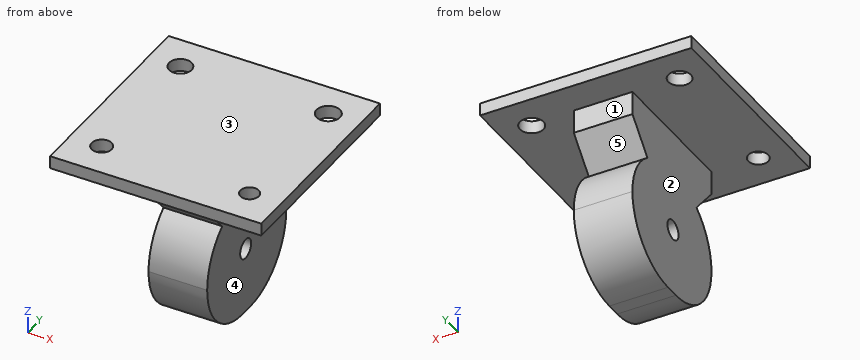
from build123d import *

# Parameters (mm, degrees)
SKETCH_W        = 50
SKETCH_H        = 50
SKETCH_R        = 2.673206
SKETCH_R_2      = 2.795993
SKETCH_R_3      = 2.184497
SKETCH_R_4      = 2.376808
PAD_DEPTH       = 3
SKETCH001_W     = 13.880783
SKETCH001_H     = 33.313887
PAD001_DEPTH    = 40
FILLET_R        = 15
POCKET_DEPTH    = 31.618891
SKETCH003_R     = 2.326985
POCKET001_DEPTH = 32.263892


with BuildPart() as part:
    # Sketch → Pad (new body)
    with BuildSketch(Plane.XY):
        Rectangle(SKETCH_W, SKETCH_H)
        with Locations((-17.5, 16.5883488719)):
            Circle(SKETCH_R, mode=Mode.SUBTRACT)
        with Locations((17.5, 16.588348)):
            Circle(SKETCH_R_2, mode=Mode.SUBTRACT)
        with Locations((17.5, -16.5883488719)):
            Circle(SKETCH_R_3, mode=Mode.SUBTRACT)
        with Locations((-17.5, -16.5883488719)):
            Circle(SKETCH_R_4, mode=Mode.SUBTRACT)
    extrude(amount=PAD_DEPTH)

    # Sketch001 (on Face9 of Pad) → Pad001 (join)
    with BuildSketch(Plane(origin=(0, 0, 0), x_dir=(1, 0, 0), z_dir=(0, 0, -1))):
        with Locations((0.3225005, -0.4243995)):
            Rectangle(SKETCH001_W, SKETCH001_H)
    extrude(amount=PAD001_DEPTH)

    # Fillet
    fillet_edges = [part.edges().sort_by_distance(p)[0] for p in [
        (0.3225, -16.232544, -40),
        (0.322501, 17.081343, -40),
    ]]
    fillet(fillet_edges, radius=FILLET_R)

    # Sketch002 (on Face1 of Fillet) → Pocket (cut, through all)
    with BuildSketch(Plane(origin=(-6.617891, 0, 0), x_dir=(0, -1, 0), z_dir=(-1, 0, 0))):
        with BuildLine():
            ThreePointArc((16.232544, -25), (14.5567914087, -18.1105565543), (9.9039532011, -12.7604468028))
            Line((9.9039532011, -12.7604468028), (16.232544, -5.5931115513))
            Line((16.232544, -5.5931115513), (16.232544, -25))
        make_face()
        with BuildLine():
            ThreePointArc((-10.7527522011, -12.7604468028), (-15.4055904087, -18.1105565543), (-17.081343, -25))
            Line((-17.081343, -5.5931115513), (-17.081343, -25))
            Line((-10.7527522011, -12.7604468028), (-17.081343, -5.5931115513))
        make_face()
    extrude(amount=-POCKET_DEPTH, mode=Mode.SUBTRACT)

    # Sketch003 (on Face18 of Pocket) → Pocket001 (cut, through all)
    with BuildSketch(Plane.YZ.offset(7.262892)):
        with Locations((0, -24.346371)):
            Circle(SKETCH003_R)
    extrude(amount=-POCKET001_DEPTH, mode=Mode.SUBTRACT)


solid = part.part
Input: part model. Units: mm. Frame: model coordinates. Face numbers are marked on the shaded views. A direction names the side the tool comes from. Round coordinates to 2 decimals unless told otherwise and drop trailing zeros. Write each loop counter-clockwise with the first axis right and the second up, starting at its lowest first coordinate (ties: lowest second). Pieces come first, ordered by that corner, then holes.
1) Cut plane B-B (y = -12.5). Return the cut outline in (x, z), then the cut area to 3 significant figures.
2) Cut plane A-A (x = 17.5). Return the cut outline in (y, z), then the cut area to 3 significant figures.
3) Draft query along Z for the marked faces 3, 4 and 5. Return one class per face: pulls with the +Z half, pulls with the -Z half, needs draft (parallel to the pull), parting line crosses it, or undercut.
4) Cut plane D-D (y = 5.5). Return the cut outline in (x, z).
5) Reachability of the marked faces 1 and 2 from +Z, -Z, +X, -X, +Y, -Y: full face, straight path, thin tool, end or side. Return the list, or none.
6) Cut plane C-C (x = -3.5). Return the cut outline in (y, z), then the cut area to 3 significant figures.
7) Contact query for flat-ended pins moving along their axis: P1, Ø10, axis at y = -4.5, z = -12, coming from the +X side; P2, Ø4.5, axis at x = -2, z = -1.5, coming from the -Y side; P3, Ø15, axis at x = -4.5, y = 11.5, coming from the -Z side; P4, Ø2, axis at x = 8.5, y = -7, coming from the -Z side. Output: stop coordinate, or through.
8) Ray query, L1, parallel to Y at x = 17.5, z = 1.75; L2, parallel to Y at x = -17.5, z = 1.1; L3, parallel to Z at x = 3.5, y = 0. Return the intervals inside material, ascending.
Geometry says:
1. outline: (-25, 0) - (-6.62, 0) - (-6.62, -9.82) - (7.26, -9.82) - (7.26, 0) - (25, 0) - (25, 3) - (-25, 3) - close; (-6.62, -34.9) - (7.26, -34.9) - (7.26, -15.1) - (-6.62, -15.1) - close
1. area: 561 mm2
2. outline: (-25, 0) - (-18.77, 0) - (-18.77, 3) - (-25, 3) - close; (-14.4, 0) - (13.79, 0) - (13.79, 3) - (-14.4, 3) - close; (19.38, 0) - (25, 0) - (25, 3) - (19.38, 3) - close
2. area: 120 mm2
3. face 3: pulls with the +Z half
3. face 4: needs draft
3. face 5: undercut
4. outline: (-25, 0) - (-6.62, 0) - (-6.62, -39.61) - (7.26, -39.61) - (7.26, 0) - (25, 0) - (25, 3) - (-25, 3) - close
5. face 1: -Z, +X, -X, +Y
5. face 2: -Z, -X, +Y, -Y
6. outline: (-25, 0) - (-16.23, 0) - (-16.23, -5.59) - (-9.9, -12.76) arc R15 ccw to (-1.23, -40) - (2.08, -40) arc R15 ccw to (10.75, -12.76) - (17.08, -5.59) - (17.08, 0) - (25, 0) - (25, 3) - (-25, 3) - close; hole circle Ø4.65 at (0, -24.35)
6. area: 1,280 mm2
7. P1: stops at x = 7.26
7. P2: stops at y = -25
7. P3: stops at z = -39.88
7. P4: stops at z = 0
8. L1: y = -25 to -18.77, -14.4 to 13.79, 19.38 to 25
8. L2: y = -25 to -18.97, -14.21 to 13.92, 19.26 to 25
8. L3: z = -40 to -26.67, -22.02 to 3
